from build123d import *

# Parameters (mm, degrees)
EXTRUDE_1_DEPTH          = 105
SKETCH_7_W               = 30.4
SKETCH_7_H               = 19
EXTRUDE_2_DEPTH          = 3
SKETCH_8_W               = 30.4
SKETCH_8_H               = 12
EXTRUDE_3_DEPTH          = 38
FILLET_1_R               = 5
CUT_EXTRUDE_1_DEPTH      = 112
CUT_EXTRUDE_2_DEPTH      = 97
CUT_EXTRUDE_4_DEPTH      = 187.349134691
CUT_EXTRUDE_4_DEPTH_BACK = 6.8
SKETCH_11_R              = 5
FILLET_3_R               = 3
SKETCH_12_R              = 2.6
CUT_EXTRUDE_5_DEPTH      = 20
CHAMFER_1_SIZE           = 3
SKETCH_13_R              = 2.9
CUT_EXTRUDE_6_DEPTH      = 187.349134691
CHAMFER_3_SIZE           = 2.5
SKETCH_16_W              = 75
SKETCH_16_H              = 48
CUT_EXTRUDE_9_DEPTH      = 187.349134691
FILLET_4_R               = 30
SKETCH_17_W              = 28
SKETCH_17_H              = 52
CUT_EXTRUDE_10_DEPTH     = 20
FILLET_5_R               = 8
SKETCH_18_W              = 8
SKETCH_18_H              = 19
EXTRUDE_4_DEPTH          = 49
CHAMFER_4_SIZE           = 50
FILLET_6_R               = 10
SKETCH_19_R              = 2.9
CUT_EXTRUDE_11_DEPTH     = 187.349134691
CHAMFER_5_SIZE           = 2.6
SKETCH_21_R              = 2.3
CUT_EXTRUDE_13_DEPTH     = 15
FILLET_7_R               = 5
CHAMFER_6_SIZE           = 0.8
SKETCH_22_W              = 8
SKETCH_22_H              = 43.683816014
EXTRUDE_5_DEPTH          = 10
FILLET_8_R               = 10


with BuildPart() as part:
    # Sketch 2 → Extrude 1 (new body)
    with BuildSketch(Plane(origin=(0, 0, 0), x_dir=(1, 0, 0), z_dir=(0, 1, 0))):
        Polygon((52.378939236, 0), (52.378939236, -103), (24.378939236, -117), (24.378939236, -135), (0, -135), (-21.621060764, -135), (-21.621060764, 0), (-8.021060764, 0), (-8.021060764, -131), (0, -131), (22.378939236, -131), (22.378939236, 0), align=None)
    extrude(amount=EXTRUDE_1_DEPTH)



with BuildPart() as body_2:
    # Sketch 7 → Extrude 2 (new body)
    with BuildSketch(Plane.XZ):
        with Locations((7.178939236, 121.5)):
            Rectangle(SKETCH_7_W, SKETCH_7_H)
    extrude(amount=-EXTRUDE_2_DEPTH)


with BuildPart() as part_1:
    add(part.part)

    add(body_2.part)  # Extrude 3 merges body 2
    # Sketch 8 → Extrude 3 (add)
    with BuildSketch(Plane(origin=(0, 3, 0), x_dir=(1, 0, 0), z_dir=(0, 1, 0))):
        with Locations((7.178939236, -125)):
            Rectangle(SKETCH_8_W, SKETCH_8_H)
    extrude(amount=EXTRUDE_3_DEPTH)

    # Fillet 1
    fillet_1_edges = [part_1.edges().sort_by_distance(p)[0] for p in [
        (7.178939236, 41, 119),
    ]]
    fillet(fillet_1_edges, radius=FILLET_1_R)

    # Sketch 3 → Cut-Extrude 1 (cut)
    with BuildSketch(Plane(origin=(0, 0, 0), x_dir=(-1, 0, 0), z_dir=(0, 0, -1))):
        Polygon((8.021060764, -1.66), (19.321060764, 3.4), (19.321060764, 5), (8.021060764, 5), align=None)
        Polygon((-33.678939236, 5), (-22.378939236, 5), (-22.378939236, -1.66), (-33.678939236, 3.4), align=None)
    extrude(amount=-CUT_EXTRUDE_1_DEPTH, mode=Mode.SUBTRACT)

    # Sketch 9 → Cut-Extrude 2 (cut)
    with BuildSketch(Plane(origin=(0, 105, 0), x_dir=(1, 0, 0), z_dir=(0, 1, 0))):
        Polygon((-21.621060764, 0), (-21.621060764, -91), (22.378939236, -91), (22.378939236, -112), (47.378939236, -99.5), (47.378939236, 0), align=None)
    extrude(amount=-CUT_EXTRUDE_2_DEPTH, mode=Mode.SUBTRACT)

    # Sketch 11 → Cut-Extrude 4 (cut, two sides: drawn at the far end of the back side and taken through both)
    with BuildSketch(Plane.ZY.offset(21.621060764).offset(-CUT_EXTRUDE_4_DEPTH_BACK)):
        with Locations(Location((98.6, 41.2, 0), (0, 0, 180))):
            Circle(SKETCH_11_R)
    extrude(amount=CUT_EXTRUDE_4_DEPTH + CUT_EXTRUDE_4_DEPTH_BACK, mode=Mode.SUBTRACT)

    # Fillet 3
    fillet_3_edges = [part_1.edges().sort_by_distance(p)[0] for p in [
        (47.378939236, 56.5, 99.5),
        (22.378939236, 56.5, 112),
        (24.378939236, 52.5, 135),
        (24.378939236, 52.5, 117),
    ]]
    fillet(fillet_3_edges, radius=FILLET_3_R)

    # Sketch 12 → Cut-Extrude 5 (cut)
    with BuildSketch(Plane.ZY.offset(21.621060764)):
        with Locations((98.6, 41.2)):
            Circle(SKETCH_12_R)
    extrude(amount=-CUT_EXTRUDE_5_DEPTH, mode=Mode.SUBTRACT)

    # Chamfer 1
    # the kernel refuses this chamfer: 3 mm, written as the material it takes off along each edge
    with BuildSketch(Plane(origin=(-14.821060764, 41.2, 98.6), x_dir=(0, 0, 1), z_dir=(0, -1, 0))) as chamfer_1_piece_1_section:
        Polygon((2.6, -CHAMFER_1_SIZE), (2.6 + CHAMFER_1_SIZE, 0), (2.6, 0), align=None)
    chamfer_1_piece_1 = revolve(axis=Axis((-14.821060764, 41.2, 98.6), (-1, 0, 0)), mode=Mode.PRIVATE)
    chamfer_1_piece_1 = chamfer_1_piece_1 & Plane(origin=(-13.01179882, 41.2, 98.6), x_dir=(0, 0, -1), z_dir=(-1, 0, 0)) * Cylinder(5, 23, mode=Mode.PRIVATE)
    add(chamfer_1_piece_1, mode=Mode.SUBTRACT)

    # Sketch 13 → Cut-Extrude 6 (cut, through all)
    with BuildSketch(Plane.ZY.offset(21.621060764)):
        with Locations((83, 46)):
            Circle(SKETCH_13_R)
        with Locations((13, 46)):
            Circle(SKETCH_13_R)
        with Locations((83, 96)):
            Circle(SKETCH_13_R)
    extrude(amount=-CUT_EXTRUDE_6_DEPTH, mode=Mode.SUBTRACT)

    # Chamfer 3
    chamfer_3_edges = [part_1.edges().sort_by_distance(p)[0] for p in [
        (47.378939236, 96, 80.1),
        (47.378939236, 46, 10.1),
        (47.378939236, 46, 80.1),
    ]]
    chamfer(chamfer_3_edges, length=CHAMFER_3_SIZE)

    # Sketch 16 → Cut-Extrude 9 (cut, through all)
    with BuildSketch(Plane.ZY.offset(21.621060764)):
        with Locations((37.5, 81)):
            Rectangle(SKETCH_16_W, SKETCH_16_H)
    extrude(amount=-CUT_EXTRUDE_9_DEPTH, mode=Mode.SUBTRACT)

    # Fillet 4
    fillet_4_edges = [part_1.edges().sort_by_distance(p)[0] for p in [
        (49.878939236, 57, 75),
    ]]
    fillet(fillet_4_edges, radius=FILLET_4_R)

    # Sketch 17 → Cut-Extrude 10 (cut)
    with BuildSketch(Plane.ZY.offset(21.621060764)):
        with Locations((105, 79)):
            Rectangle(SKETCH_17_W, SKETCH_17_H)
    extrude(amount=-CUT_EXTRUDE_10_DEPTH, mode=Mode.SUBTRACT)

    # Fillet 5
    fillet_5_edges = [part_1.edges().sort_by_distance(p)[0] for p in [
        (-14.821060764, 53, 91),
        (-14.821060764, 53, 119),
    ]]
    fillet(fillet_5_edges, radius=FILLET_5_R)

    # Sketch 18 → Extrude 4 (add)
    with BuildSketch(Plane(origin=(0, 8, 0), x_dir=(1, 0, 0), z_dir=(0, 1, 0))):
        with Locations((-17.621060764, -9.5)):
            Rectangle(SKETCH_18_W, SKETCH_18_H)
    extrude(amount=EXTRUDE_4_DEPTH)

    # Chamfer 4
    # the kernel refuses this chamfer: 50 mm, written as the material it adds along each edge
    with BuildSketch(Plane(origin=(-13.621060764, 8, 19), x_dir=(0, 0.9996219169112966, -0.027495876610586386), z_dir=(-1, 0, 0))) as chamfer_4_piece_1_section:
        Polygon((CHAMFER_4_SIZE * 0.999621916911, -CHAMFER_4_SIZE * 0.0274958766106), (-CHAMFER_4_SIZE * 0.0274958766106, -CHAMFER_4_SIZE * 0.999621916911), (0, 0), align=None)
    chamfer_4_piece_1 = extrude(amount=8, mode=Mode.PRIVATE)
    chamfer_4_piece_1 = split(chamfer_4_piece_1, bisect_by=Plane(origin=(-17.621060764, 57, 35.555220818), z_dir=(0, -1, 0)), keep=Keep.TOP, mode=Mode.PRIVATE)
    add(chamfer_4_piece_1)

    # Fillet 6
    fillet_6_edges = [part_1.edges().sort_by_distance(p)[0] for p in [
        (49.878939236, 57, 0),
        (-17.621060764, 57, 0),
    ]]
    fillet(fillet_6_edges, radius=FILLET_6_R)

    # Sketch 19 → Cut-Extrude 11 (cut, through all)
    with BuildSketch(Plane(origin=(52.378939236, 0, 0), x_dir=(0, 0, -1), z_dir=(1, 0, 0))):
        with Locations(Location((-13, 46, 0), (0, 0, 180))):
            Circle(SKETCH_19_R)
    extrude(amount=-CUT_EXTRUDE_11_DEPTH, mode=Mode.SUBTRACT)

    # Chamfer 5
    chamfer_5_edges = [part_1.edges().sort_by_distance(p)[0] for p in [
        (-21.621060764, 46, 10.1),
    ]]
    chamfer(chamfer_5_edges, length=CHAMFER_5_SIZE)

    # Sketch 21 → Cut-Extrude 13 (cut)
    with BuildSketch(Plane.ZY.offset(21.621060764)):
        with Locations((125, 30)):
            Circle(SKETCH_21_R)
        with Locations((125, 90)):
            Circle(SKETCH_21_R)
    extrude(amount=-CUT_EXTRUDE_13_DEPTH, mode=Mode.SUBTRACT)

    # Fillet 7
    fillet_7_edges = [part_1.edges().sort_by_distance(p)[0] for p in [
        (49.878939236, 105, 75),
        (-14.821060764, 105, 119),
    ]]
    fillet(fillet_7_edges, radius=FILLET_7_R)

    # Chamfer 6
    chamfer_6_edges = [part_1.edges().sort_by_distance(p)[0] for p in [
        (-21.621060764, 41.2, 103.6),
        (-21.621060764, 30, 122.7),
        (-21.621060764, 90, 122.7),
    ]]
    chamfer(chamfer_6_edges, length=CHAMFER_6_SIZE)

    # Sketch 22 → Extrude 5 (add)
    with BuildSketch(Plane(origin=(0, 8, 0), x_dir=(1, 0, 0), z_dir=(0, 1, 0))):
        with Locations((-17.621060764, -69.158091993)):
            Rectangle(SKETCH_22_W, SKETCH_22_H)
    extrude(amount=EXTRUDE_5_DEPTH)

    # Fillet 8
    fillet_8_edges = [part_1.edges().sort_by_distance(p)[0] for p in [
        (-17.621060764, 57, 20),
    ]]
    fillet(fillet_8_edges, radius=FILLET_8_R)


solid = part_1.part
Source: CAD feature listing. Evaluate the final solid. Frame: model axes, mm. A direction names the side the tool comes from. Give positions to 0.01 mm unless a question says otherwise; leave off trailing zeros. Write each loop counter-clockwise with the first axis right and the second up, starting at its lowest first coordinate (ties: lowest second). Pieces come first, ordered by that corner, then holes. Notation, with made-up numbers: (68.25, -20) -> (75.25, -20) arc R28 cw to (75.25, 9) -> close; hole circle Ø9 at (77.5, 79.25). An arc over 180 degrees is marked (long way). Return JSON: item names as keys, results as strings. Group by question number.
1. Section B-B, the plane y = 30. Output: boundary loops of the cut face in (x, z).
2. Pin query (flat end, axial travel): pin 1 Ø9.5 at (y, z) = (46, 13) entering from -X; pin 2 Ø7.5 at (y, z) = (46, 13) entering from -X; pin 3 Ø3.5 at (x, z) = (26, 32.5) entering from -Y; pin 4 Ø4.5 at (x, z) = (-11, 55) entering from +Y. Return the tip coordinate at first contact, or that it passes through.
3. Access query for faces 1 (the face through (-15, 104, 121)), 2 (the face through (-14, 5, 55)), 3 (the face through (49.758, 48.996, 12.607)), 4 (the face through (7, 19, 119)). Directions: +Z, -Z, +X, -X, +Y, -Y. A direction counts if a zero-diameter tool reaches every point of the face in a straight line with its end or side. Return the directions, or none.
4. Material intervals for line 1 (Y direction, x = 50.7, z = 83); line 2 (X direction, y = 25, z = 51.5); line 3 (X direction, y = 50, z = 94), sorted ascending. Write a range as from..to.
5. Section C-C, the plane x = -10. Output: boundary loops of the cut face in (y, z), then the cut area to 3 significant figures.
6. Mould query, pull axis Z, two halves, no side actions, for faces 5 (the face through (-15, 80, 119)), 6 (the face through (-13.621, 27, 36)), 7 (the face through (-14.726, 55.406, 116.719)). Classes: +Z half, -Z half, draft (parallel to the pull), parting line (faces both ways), or undercut.
7. Section A-A, the plane z = 13. Count the separate pieces of the cut face and the enclosed holes in it, then the cut area to 3 significant figures.
8. Section D-D, the plane z = 41. Output: boundary loops of the cut face in (x, y), then the cut area to 3 significant figures.
Determined:
{
 "1": {"outline": "(-21.62, 0) -> (-13.62, 0) -> (-13.62, 47) -> (-21.62, 47) -> close; (-21.62, 91) -> (-8.02, 91) -> (-8.02, 119) -> (22.38, 119) -> (22.38, 113.85) arc R3 ccw to (24.04, 111.17) -> (45.72, 100.33) arc R3 cw to (47.38, 97.65) -> (47.38, 0) -> (52.38, 0) -> (52.38, 103) -> (26.04, 116.17) arc R3 cw to (24.38, 118.85) -> (24.38, 132) arc R3 ccw to (21.38, 135) -> (-21.62, 135) -> (-21.62, 128.1) -> (-20.82, 127.3) -> (-6.62, 127.3) -> (-6.62, 122.7) -> (-20.82, 122.7) -> (-21.62, 121.9) -> close"},
 "2": {"pin 1": "stops at x = -20.87", "pin 2": "stops at x = -19.87", "pin 3": "stops at y = 0", "pin 4": "stops at y = 8"},
 "3": {"face 1": "-Z, -X, +Y", "face 2": "-Z", "face 3": "none", "face 4": "-Z, +Y"},
 "4": {"line 1": "y = 0..43.1, 48.9..93.1, 98.9..105", "line 2": "x = -21.62..-13.62, 47.38..52.38", "line 3": "x = -21.62..-8.02, 47.38..52.38"},
 "5": {"outline": "(0, 112) -> (5, 112) -> (5, 0) -> (8, 0) -> (8, 91) -> (45, 91) arc R8 ccw to (53, 99) -> (53, 111) arc R8 cw to (61, 119) -> (100, 119) arc R5 ccw to (105, 124) -> (105, 135) -> (0, 135) -> close; hole circle Ø4.6 at (30, 125); hole circle Ø5.2 at (41.2, 98.6); hole circle Ø4.6 at (90, 125)", "area": "3,270 mm2"},
 "6": {"face 5": "-Z half", "face 6": "draft", "face 7": "undercut"},
 "7": {"separate pieces": "4", "enclosed holes": "0", "area": "810 mm2"},
 "8": {"outline": "(-21.62, 0) -> (-11.73, 0) -> (-19.32, 3.4) -> (-19.32, 5) -> (-8.02, 5) -> (-8.02, 8) -> (-13.62, 8) -> (-13.62, 36) -> (-21.62, 36) -> close; (22.38, 5) -> (33.68, 5) -> (33.68, 3.4) -> (26.09, 0) -> (52.38, 0) -> (52.38, 57) -> (47.38, 57) -> (47.38, 8) -> (22.38, 8) -> close", "area": "731 mm2"}
}
